For this review, take the finished solid that the model builds, in its own axes (mm). Face numbers are marked on the shaded views. A direction names the side the tool comes from. Round coordinates to 2 decimals unless told otherwise and drop trailing zeros. Write each loop counter-clockwise with the first axis right and the second up, starting at its lowest first coordinate (ties: lowest second). Pieces come first, ordered by that corner, then holes. Notation, with made-up numbers: (44.5, 26.25) -> (57.5, 26.25) arc R14 cw to (57.5, 43.25) -> close; hole circle Ø7 at (45, 4). An arc over 180 degrees is marked (long way). Answer in a Markdown table with one row per item.
from build123d import *

# Parameters (mm, degrees)
SKETCH_3_W          = 20
SKETCH_3_H          = 59
EXTRUDE_2_DEPTH     = 6
SKETCH_10_R         = 2.2
CUT_EXTRUDE_3_DEPTH = 61.141499815
SKETCH_11_W         = 20
SKETCH_11_H         = 22
EXTRUDE_5_DEPTH     = 6
SKETCH_9_W          = 20
SKETCH_9_H          = 7.4
EXTRUDE_4_DEPTH     = 0.4
SKETCH_13_R         = 2.6
CUT_EXTRUDE_4_DEPTH = 70.722019477
EXTRUDE_6_DEPTH     = 4


with BuildPart() as part:
    # Эскиз3 → Бобышка-Вытянуть2 (new body)
    with BuildSketch(Plane.XY):
        with Locations((0, 29.5)):
            Rectangle(SKETCH_3_W, SKETCH_3_H)
    extrude(amount=EXTRUDE_2_DEPTH)

    # Эскиз10 → Вырез-Вытянуть3 (cut, through all)
    with BuildSketch(Plane(origin=(0, 0, 0), x_dir=(-1, 0, 0), z_dir=(0, 0, -1))):
        with Locations((0, 17.5)):
            Circle(SKETCH_10_R)
    extrude(amount=-CUT_EXTRUDE_3_DEPTH, mode=Mode.SUBTRACT)

    # Эскиз11 → Бобышка-Вытянуть5 (add)
    with BuildSketch(Plane(origin=(0, 59, 0), x_dir=(1, 0, 0), z_dir=(0, 1, 0))):
        with Locations((0, -11)):
            Rectangle(SKETCH_11_W, SKETCH_11_H)
    extrude(amount=EXTRUDE_5_DEPTH)

    # Эскиз9 → Бобышка-Вытянуть4 (add)
    with BuildSketch(Plane(origin=(0, 65, -43.4), x_dir=(1, 0, 0), z_dir=(0, -1, 0))):
        with Locations((0, 55.4)):
            Rectangle(SKETCH_9_W, SKETCH_9_H)
    extrude(amount=-EXTRUDE_4_DEPTH)

    # Эскиз13 → Вырез-Вытянуть4 (cut, through all)
    with BuildSketch(Plane(origin=(0, 65.4, 0), x_dir=(1, 0, 0), z_dir=(0, 1, 0))):
        with Locations(Location((0, -12, 0), (0, 0, 270))):
            Circle(SKETCH_13_R)
    extrude(amount=-CUT_EXTRUDE_4_DEPTH, mode=Mode.SUBTRACT)

    # Эскиз17 → Бобышка-Вытянуть6 (add)
    with BuildSketch(Plane.ZY.offset(10)):
        Polygon((22, 59), (6, 59), (6, 0), align=None)
    extrude_6 = extrude(amount=-EXTRUDE_6_DEPTH)

    # Зеркальное отражение1: Бобышка-Вытянуть6 across plane
    add(extrude_6.mirror(Plane(origin=(0, 0, 0), x_dir=(0, 0, 1), z_dir=(1, 0, 0))))


solid = part.part
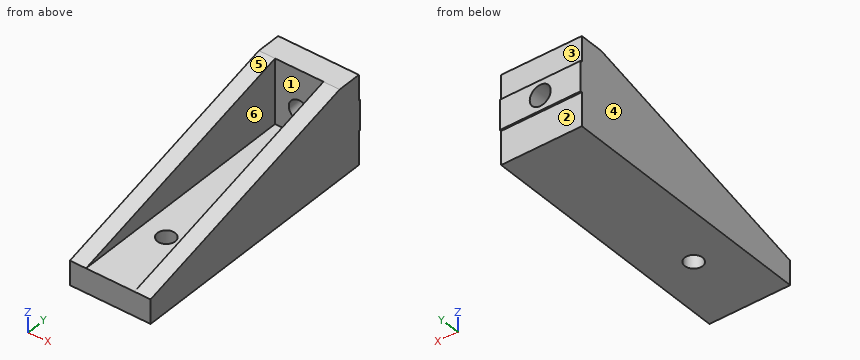
1) For the marked faces 1, 2 and 3, list the 3-axis set-ups (+Z, -Z, +X, -X, +Y, -Y) from which the entire face can be reached by the end or side of a thin tool; tool diameter is ignored.
Solved:
| item | result |
|---|---|
| face 1 | +Z, -Y |
| face 2 | -Z, +X, -X, +Y |
| face 3 | +Z, +X, -X, +Y |
2) For line 1 (X direction, y = 62.25, z = 12); line 2 (X direction, y = 33, z = 8.25); line 3 (Y direction, x = 8.5, z = 4), list the stretches that pass through material, from the lowest coordinate up. Write a range as [from, to].
Solved:
| item | result |
|---|---|
| line 1 | [-10, -2.6], [2.6, 10] |
| line 2 | [-10, -6], [6, 10] |
| line 3 | [0, 65] |
3) Consider section A-A on x = 0. State the section outline as (y, z) points, then the cut area to 3 significant figures.
Solved:
| item | result |
|---|---|
| outline | (0, 0) -> (15.3, 0) -> (15.3, 6) -> (0, 6) -> close; (19.7, 0) -> (65, 0) -> (65, 8.3) -> (65.4, 8.3) -> (65.4, 9.4) -> (59, 9.4) -> (59, 6) -> (19.7, 6) -> close; (59, 14.6) -> (65.4, 14.6) -> (65.4, 15.7) -> (65, 15.7) -> (65, 22) -> (59, 22) -> close |
| area | 429 mm² |
4) Consider section C-C on y = 17.5. State the section outline as (x, z) points.
Solved:
| item | result |
|---|---|
| outline | (-10, 0) -> (-2.2, 0) -> (-2.2, 6) -> (-6, 6) -> (-6, 10.75) -> (-10, 10.75) -> close; (2.2, 0) -> (10, 0) -> (10, 10.75) -> (6, 10.75) -> (6, 6) -> (2.2, 6) -> close |
5) Mouldability with a two-part tool opening along X and no side actions: class the marked faces 4, 5 and 6 as pulls with the +X half, pulls with the -X half, needs draft (parallel to the pull), parting line crosses it, or undercut.
Solved:
| item | result |
|---|---|
| face 4 | pulls with the -X half |
| face 5 | needs draft |
| face 6 | undercut |
6) Clearance check with flat-ended pins moving along their axes: pin 1 Ø4 at (x, z) = (-7.5, 4.5) entering from +Y; pin 2 Ø12 at (x, z) = (-4, 8.5) entering from -Y; pin 3 Ø6 at (x, z) = (0, 12) entering from -Y; pin 4 Ø3.5 at (x, y) = (3, 41) entering from +Z. State where each tip first meets the part, or that it passes through.
Solved:
| item | result |
|---|---|
| pin 1 | y = 65 |
| pin 2 | y = 0 |
| pin 3 | y = 59 |
| pin 4 | z = 6 |
7) Consider section D-D on x = -4.5. State the section outline as (y, z) points.
Solved:
| item | result |
|---|---|
| outline | (0, 0) -> (65, 0) -> (65, 8.3) -> (65.4, 8.3) -> (65.4, 15.7) -> (65, 15.7) -> (65, 22) -> (59, 22) -> (59, 6) -> (0, 6) -> close |
8) Consider section B-B on z = 11. State the section outline as (x, y) points, then the cut area to 3 significant figures.
Solved:
| item | result |
|---|---|
| outline | (-10, 18.44) -> (-6, 18.44) -> (-6, 59) -> (-2.4, 59) -> (-2.4, 65.4) -> (-10, 65.4) -> close; (2.4, 59) -> (6, 59) -> (6, 18.44) -> (10, 18.44) -> (10, 65.4) -> (2.4, 65.4) -> close |
| area | 422 mm² |
